```python
from build123d import *

# Parameters (mm, degrees)
F1_DEPTH = 50.8
F0_W     = 6.35
F0_H     = 11.938
F2_DEPTH = 50.8
F0_W_2   = 44.45
F3_DEPTH = 6.35


with BuildPart() as f1:
    # F0 (on Front) → F1 (new body)
    with BuildSketch(Plane.XZ):
        Polygon((6.35, 0), (0, 0), (0, -131.7625), (50.8, -131.7625), (50.8, 0), align=None)
    extrude(amount=F1_DEPTH)

    # F0 (on Front) → F2 (join, through all)
    with BuildSketch(Plane.XZ):
        with Locations((3.175, 5.969)):
            Rectangle(F0_W, F0_H)
    extrude(amount=F2_DEPTH)

    # F0 (on Front) → F3 (join)
    with BuildSketch(Plane.XZ):
        with Locations((28.575, 5.969)):
            Rectangle(F0_W_2, F0_H)
    extrude(amount=F3_DEPTH)


solid = f1.part
```
Here's how the part is built. I have some questions about the finished solid (model axes, mm). A direction names the side the tool comes from. Coordinates: 2 decimals unless noted, no trailing zeros. Loops run counter-clockwise (first coordinate to the right, second up) from the corner with the lowest first, then second, coordinate; pieces in that order, holes last. Notation, with made-up numbers: M -23.5,74 L -0.5,74 A13 cw -0.5,83 Z; hole C 59,50.25 d7. An arc over 180 degrees is marked long. One line per item, written item: value.
1. On a 3-axis mill with a long thin cutter (end or side, diameter ignored), from which of +Z, -Z, +X, -X, +Y, -Y can I reach the whole of each face in a straight line? I mean faces 1 (the flat face through (25, -25, -131.762)), 2 (the flat face through (29, -28, 0)). Say none if no direction works.
Geometry says:
face 1: -Z, +X, -X, +Y, -Y
face 2: +Z, +X, -Y
2. Imagine slicing it at A-A (y = -17). List the corners of the cut face in (x, z) for me.
Geometry says:
outline: M 0,-131.76 L 50.8,-131.76 L 50.8,0 L 6.35,0 L 6.35,11.94 L 0,11.94 Z
3. Please list where this line runs through material, in increasing order: probe 1 along Z at (x, y) = (8, -16).
Geometry says:
probe 1: z = -131.76 to 0
4. Will these pins go through, and if not, where does the flat tip stop? pin 1 Ø6 at (x, z) = (34, 6.5) entering from -Y; pin 2 Ø13.5 at (x, y) = (18, -39) entering from +Z.
Geometry says:
pin 1: stops at y = -6.35
pin 2: stops at z = 0
5. Imagine slicing it at B-B (x = 13.5). List the corners of the cut face in (y, z) for me, and give its area (3 significant figures).
Geometry says:
outline: M -50.8,-131.76 L 0,-131.76 L 0,11.94 L -6.35,11.94 L -6.35,0 L -50.8,0 Z
area: 6,770 mm2
